from build123d import *

# Parameters (mm, degrees)
F1_DEPTH = 63.5
F2_DEPTH = 25.4
F3_DEPTH = 7.9375
F5_R     = 6.35


with BuildPart() as f1:
    # F0 (on Front) → F1 (new body, symmetric)
    with BuildSketch(Plane.XZ):
        Polygon((22.225, 9.525), (-41.275, 9.525), (-41.275, -9.525), (41.275, -9.525), (41.275, 9.525), align=None)
    extrude(amount=F1_DEPTH, both=True)

    # F0 (on Front) → F2 (join, symmetric)
    with BuildSketch(Plane.XZ):
        with BuildLine():
            Line((22.225, 27.0002), (22.225, 9.525))
            Line((22.225, 9.525), (41.275, 9.525))
            Line((41.275, 9.525), (41.275, 27.0002))
            ThreePointArc((41.275, 27.0002), (45.9246798487, 38.2255201513), (57.15, 42.8752))
            Line((57.15, 42.8752), (60.325, 42.8752))
            Line((60.325, 42.8752), (60.325, 61.9252))
            Line((60.325, 61.9252), (57.15, 61.9252))
            ThreePointArc((57.15, 61.9252), (32.4542956671, 51.6959043329), (22.225, 27.0002))
        make_face()
        Polygon((85.725, 61.9252), (60.325, 61.9252), (60.325, 42.8752), (85.725, 42.8752), (85.725, 52.3875), align=None)
    extrude(amount=F2_DEPTH, both=True)

    # F0 (on Front) → F3 (join, symmetric)
    with BuildSketch(Plane.XZ):
        with BuildLine():
            add(Edge.make_bspline(
                [(-41.275, 9.525), (-41.5751747787, 48.5781729221), (22.9490175843, 63.0326196551), (57.15, 61.9252)],
                knots=[0, 0, 0, 0, 111.5045361635, 111.5045361635, 111.5045361635, 111.5045361635], degree=3))
            Line((-41.275, 9.525), (22.225, 9.525))
            Line((22.225, 9.525), (22.225, 27.0002))
            ThreePointArc((22.225, 27.0002), (32.4542956671, 51.6959043329), (57.15, 61.9252))
        make_face()
    extrude(amount=F3_DEPTH, both=True)

    # F0 (on Front) → F4 (revolve)
    with BuildSketch(Plane.XZ):
        Polygon((85.725, 66.675), (85.725, 61.9252), (85.725, 52.3875), (85.725, 42.8752), (85.725, 38.1), (111.125, 38.1), (111.125, 66.675), align=None)
    revolve(axis=Axis((85.725, 0, 21.2952332962), (0, 0, -1)))

    # F5
    f5_edges = [f1.edges().sort_by_distance(p)[0] for p in [
        (41.275, -63.5, 0),
        (-41.275, -63.5, 0),
        (-41.275, 63.5, 0),
        (41.275, 63.5, 0),
    ]]
    fillet(f5_edges, radius=F5_R)


solid = f1.part
Design review of the part built by this model. Coordinates are the model's own, in mm. A direction names the side the tool comes from. Give positions to 0.01 mm unless a question says otherwise; leave off trailing zeros. Write each loop counter-clockwise with the first axis right and the second up, starting at its lowest first coordinate (ties: lowest second). Pieces come first, ordered by that corner, then holes. Notation, with made-up numbers: M -19.75,-37 L -15.75,-37 A25 ccw -15.75,-17 Z; hole C -14.75,-38.5 d8. An arc over 180 degrees is marked long. Answer as a JSON object with one key per item and string values. Group by question number.
1) We need section B-B (y = 44). Give the boundary of the cut face in (x, z) (3 decimals), and give its area (3 significant figures).
2) For line 1 along X through (y, z) = (-31.5, 0.5) (3 decimals); line 2 along Y through (x, z) = (-6, 42); line 3 along X through (y, z) = (-20, 13) (3 decimals), list the stretches that pass through material, from the lowest coordinate up.
3) Mouldability with a two-part tool opening along X and no side actions: class faces 6 (the face through (41.275, -1, 4)), 7 (the face through (-2, 7.938, 31)), 8 (the face through (60, 2, 42.875)) as released by +X, released by -X, zero draft, split by the parting line, or undercut.
4) We need section A-A (y = -10.5). Give the boundary of the cut face in (x, z) (3 decimals), and give its area (3 significant figures).
5) Tool access review of faces 1 (the face through (46, 25.4, 42)), 2 (the face through (46, -25.4, 42)), 3 (the face through (32.73, 16.55, 51.97)), 4 (the face through (22.225, -17, 18)), 5 (the face through (45.8, -0.4, 38.1)): name each direction out of +Z, -Z, +X, -X, +Y, -Y from which nothing blocks a thin tool from reaching the whole face with its end or side.
6) Clearance check with flat-ended pins moving along their axes: pin 1 Ø16.5 at (x, y) = (10, 26.5) entering from +Z (3 decimals); pin 2 Ø5 at (x, z) = (-3, 43) entering from +Y; pin 3 Ø18.5 at (y, z) = (24.5, 9) entering from +X (3 decimals). State where each tip first meets the part, or that it passes through.
Answer key:
{
 "1": {"outline": "M -41.275,-9.525 L 41.275,-9.525 L 41.275,9.525 L -41.275,9.525 Z", "area": "1,570 mm²"},
 "2": {"line 1": "x = -41.275 to 41.275", "line 2": "y = -7.94 to 7.94", "line 3": "x = 22.225 to 41.275"},
 "3": {"face 6": "released by +X", "face 7": "zero draft", "face 8": "undercut"},
 "4": {"outline": "M -41.275,-9.525 L 41.275,-9.525 L 41.275,27 A15.875 cw 57.15,42.875 L 62.597,42.875 L 62.597,38.1 L 108.853,38.1 L 108.853,66.675 L 62.597,66.675 L 62.597,61.925 L 57.15,61.925 A34.925 ccw 22.225,27 L 22.225,9.525 L -41.275,9.525 Z", "area": "4,090 mm²"},
 "5": {"face 1": "+Z, +X, -X, +Y", "face 2": "+Z, +X, -X, -Y", "face 3": "+Z, -X, +Y", "face 4": "+Z, -X, -Y", "face 5": "-Z, +Y, -Y"},
 "6": {"pin 1": "stops at z = 9.525", "pin 2": "stops at y = 7.94", "pin 3": "stops at x = 41.275"}
}
